Autodesk Fusion 360 part; units mm, degrees
sketch "Sketch1" plane through (0, 0, 0) normal (0, 1, 0) x (1, 0, 0)
  circle A0 centre (0, 0) radius 4.5
  dimension "d1" = 9
extrude "Extrude1" add sketch "Sketch1" along normal blind 1
sketch "Sketch2" plane through (0, 1, 0) normal (0, 1, 0) x (-1, 0, 0)
  circle A0 centre (0, 0) radius 4.5
  circle A1 centre (0, 0) radius 3.048
  dimension "d4" = 6.096
extrude "Extrude2" add sketch "Sketch2" along normal blind 4 contours A1
sketch "Sketch3" plane through (0, 0, 0) normal (0, -1, 0) x (1, 0, 0)
  circle A0 centre (0, 0) radius 4.5
  circle A1 centre (0, 0) radius 1.778
  dimension "d7" = 3.556
extrude "Extrude3" cut sketch "Sketch3" against normal blind 4 contours A1
Input: part model. Units: mm. Frame: model coordinates. Round coordinates to 2 decimals unless told otherwise and drop trailing zeros. Loops run counter-clockwise (first coordinate to the right, second up) from the corner with the lowest first, then second, coordinate; pieces in that order, holes last. Notation, with made-up numbers: M 57.5,36.25 L 86.5,36.25 A30 cw 86.5,66.25 Z; hole C 14,75.5 d6. An arc over 180 degrees is marked long. Answer in a Markdown table with one row per item. Add a question column.
1. Contact query for flat-ended pins moving along their axis: pin 1 (1.5 mm diameter, centred on x = 1.5, y = 4.5, fed in from -Z); pin 2 (2 mm diameter, centred on x = 0, z = 0, fed in from -Y); pin 3 (1 mm diameter, centred on x = 3, y = 4, fed in from +Z). Output: stop coordinate, or through.
2. Section B-B (x = 0). Output: boundary loops of the cut face in (y, z).
3. Section A-A (z = 0). Output: boundary loops of the cut face in (x, y), and give its area (3 significant figures).
4. Section C-C (y = 2). Output: boundary loops of the cut face in (x, z).
5. Mould query, pull axis X, two halves, no side actions, for faces 1 (the face through (-0.385, 1.972, -1.736)), 2 (the face through (0, 4, 0)), 3 (the face through (0.4, 2.97, -3.02)), 4 (the face through (0, 0, 2)). Classes: released by +X, released by -X, zero draft, split by the parting line, or undercut.
6. Ray query, probe 1 along Z at (x, y) = (0, 1.45); probe 2 along Z at (x, y) = (0, 0.9); probe 3 along Y at (x, z) = (-1.25, -0.75). Return the intervals inside material, ascending.
7. Section D-D (y = 4.15). Output: boundary loops of the cut face in (x, z).
Values follow:
| question | item | result |
|---|---|---|
| 1 | pin 1 | z = -2.95 |
| 1 | pin 2 | y = 4 |
| 1 | pin 3 | z = 1.74 |
| 2 | outline | M 0,-4.5 L 1,-4.5 L 1,-3.05 L 5,-3.05 L 5,3.05 L 1,3.05 L 1,4.5 L 0,4.5 L 0,1.78 L 4,1.78 L 4,-1.78 L 0,-1.78 Z |
| 3 | outline | M -4.5,0 L -1.78,0 L -1.78,4 L 1.78,4 L 1.78,0 L 4.5,0 L 4.5,1 L 3.05,1 L 3.05,5 L -3.05,5 L -3.05,1 L -4.5,1 Z |
| 3 | area | 19.2 mm^2 |
| 4 | outline | C 0,0 d6.1; hole C 0,0 d3.56 |
| 5 | face 1 | undercut |
| 5 | face 2 | undercut |
| 5 | face 3 | split by the parting line |
| 5 | face 4 | zero draft |
| 6 | probe 1 | -3.05 to -1.78, 1.78 to 3.05 |
| 6 | probe 2 | -4.5 to -1.78, 1.78 to 4.5 |
| 6 | probe 3 | 4 to 5 |
| 7 | outline | C 0,0 d6.1 |
